```python
from build123d import *

# Parameters (mm, degrees)
SKETCH1_W                                           = 260
SKETCH1_H                                           = 190
BOSS_EXTRUDE1_DEPTH                                 = 40
SKETCH2_R                                           = 15
CUT_EXTRUDE1_DEPTH                                  = 166.90660023
SKETCH3_R                                           = 5.05
CUT_EXTRUDE2_DEPTH                                  = 166.90660023
SKETCH4_R                                           = 9.770548986
CUT_EXTRUDE3_DEPTH                                  = 166.90660023
CBORE_FOR_M8_HEX_SOCKET_HEAD_CAP_SCREW1_D           = 8.4
CBORE_FOR_M8_HEX_SOCKET_HEAD_CAP_SCREW1_CBORE_D     = 15
CBORE_FOR_M8_HEX_SOCKET_HEAD_CAP_SCREW1_CBORE_DEPTH = 8.6
F_8_0MM_DOWEL_HOLE1_D                               = 8
F_10_0MM_DOWEL_HOLE1_D                              = 10
SKETCH15_R                                          = 8.5
CUT_EXTRUDE4_DEPTH                                  = 31.9


with BuildPart() as part:
    # Sketch1 → Boss-Extrude1 (new body)
    with BuildSketch(Plane(origin=(0, 0, 0), x_dir=(1, 0, 0), z_dir=(0, 1, 0))):
        Rectangle(SKETCH1_W, SKETCH1_H)
    extrude(amount=-BOSS_EXTRUDE1_DEPTH)

    # Sketch2 → Cut-Extrude1 (cut, through all)
    with BuildSketch(Plane(origin=(0, 0, 0), x_dir=(1, 0, 0), z_dir=(0, 1, 0))):
        with Locations(Location((-90, 55, 0), (0, 0, 270))):
            Circle(SKETCH2_R)
        with Locations(Location((90, 55, 0), (0, 0, 270))):
            Circle(SKETCH2_R)
    extrude(amount=-CUT_EXTRUDE1_DEPTH, mode=Mode.SUBTRACT)

    # Sketch3 → Cut-Extrude2 (cut, through all)
    with BuildSketch(Plane.XZ.offset(40)):
        with Locations(Location((-55, 70, 0), (0, 0, 270))):
            Circle(SKETCH3_R)
        with Locations(Location((55, 70, 0), (0, 0, 270))):
            Circle(SKETCH3_R)
        with Locations(Location((55, -5, 0), (0, 0, 270))):
            Circle(SKETCH3_R)
        with Locations(Location((-55, -5, 0), (0, 0, 270))):
            Circle(SKETCH3_R)
    extrude(amount=-CUT_EXTRUDE2_DEPTH, mode=Mode.SUBTRACT)

    # Sketch4 → Cut-Extrude3 (cut, through all)
    with BuildSketch(Plane.XZ.offset(40)):
        with Locations(Location((0, 32.5, 0), (0, 0, 270))):
            Circle(SKETCH4_R)
    extrude(amount=-CUT_EXTRUDE3_DEPTH, mode=Mode.SUBTRACT)

    # CBORE for M8 Hex Socket Head Cap Screw1 (through all)
    with Locations(Plane(origin=(0, -40, 0), x_dir=(-1, 0, 0), z_dir=(0, -1, 0))):
        with Locations((-49, -11.95), (-49, -53.05), (49, -53.05), (49, -11.95)):
            CounterBoreHole(CBORE_FOR_M8_HEX_SOCKET_HEAD_CAP_SCREW1_D / 2, CBORE_FOR_M8_HEX_SOCKET_HEAD_CAP_SCREW1_CBORE_D / 2, CBORE_FOR_M8_HEX_SOCKET_HEAD_CAP_SCREW1_CBORE_DEPTH)

    # Ø8.0mm Dowel Hole1 (through all)
    with Locations(Plane(origin=(0, -40, 0), x_dir=(-1, 0, 0), z_dir=(0, -1, 0))):
        with Locations((-49, -32.5), (49, -32.5)):
            Hole(F_8_0MM_DOWEL_HOLE1_D / 2)

    # Ø10.0mm Dowel Hole1 (through all)
    with Locations(Plane(origin=(0, -40, 0), x_dir=(-1, 0, 0), z_dir=(0, -1, 0))):
        with Locations((-100, 17.5), (-100, -82.5), (100, -82.5), (100, 17.5)):
            Hole(F_10_0MM_DOWEL_HOLE1_D / 2)

    # Sketch15 → Cut-Extrude4 (cut)
    with BuildSketch(Plane.XZ.offset(40)):
        with Locations(Location((-100, 82.5, 0), (0, 0, 270))):
            Circle(SKETCH15_R)
        with Locations(Location((100, 82.5, 0), (0, 0, 270))):
            Circle(SKETCH15_R)
        with Locations(Location((100, -17.5, 0), (0, 0, 270))):
            Circle(SKETCH15_R)
        with Locations(Location((-100, -17.5, 0), (0, 0, 270))):
            Circle(SKETCH15_R)
    extrude(amount=-CUT_EXTRUDE4_DEPTH, mode=Mode.SUBTRACT)


solid = part.part
```
Build history of the part. All positions in model axes, mm. A direction names the side the tool comes from. Give positions to 0.01 mm unless a question says otherwise; leave off trailing zeros. Order: outer loops, then holes, each group sorted by start corner. A loop starts at its lowest first (then second) coordinate and runs counter-clockwise, first axis right, second up. Notation, with made-up numbers: M 76,9.25 L 84,9.25 A11 ccw 84,30.25 Z; hole C 28,-39 d9. An arc over 180 degrees is marked long. Return JSON: item names as keys, results as strings.
Q1. Wall check: probe 1 along Z at (x, y) = (49, -19.5); probe 2 along X at (y, z) = (-34, 53); probe 3 along X at (y, z) = (-19, 32). Give the ranges that are in metal, low to high. Write a range as from..to.
Answer list:
{"probe 1": "z = -95..7.75, 16.15..28.5, 36.5..48.85, 57.25..95", "probe 2": "x = -130..-56.5, -41.5..41.5, 56.5..130", "probe 3": "x = -130..-52.97, -45.03..-9.76, 9.76..45.03, 52.97..130"}
Q2. Flat gauge pins, fed straight in: pin 1 (7 mm diameter, centred on x = 49, z = 32.5, fed in from +Y); pin 2 (13.5 mm diameter, centred on x = -100, z = -17.5, fed in from -Y); pin 3 (12 mm diameter, centred on x = 48.5, z = 52, fed in from -Y). Where does each tip first touch, or does it go through?
Answer list:
{"pin 1": "passes through", "pin 2": "stops at y = -8.1", "pin 3": "stops at y = -31.4"}
Q3. Band-saw the part on D-D (z = -17.5). Give the cut face in (x, y), then the cut area to 3 significant figures.
Answer list:
{"outline": "M -130,-40 L -108.5,-40 L -108.5,-8.1 L -105,-8.1 L -105,0 L -130,0 Z; M -95,-8.1 L -91.5,-8.1 L -91.5,-40 L 91.5,-40 L 91.5,-8.1 L 95,-8.1 L 95,0 L -95,0 Z; M 105,-8.1 L 108.5,-8.1 L 108.5,-40 L 130,-40 L 130,0 L 105,0 Z", "area": "9,150 mm^2"}
Q4. Band-saw the part on C-C (x = 100). Give the cut face in (y, z).
Answer list:
{"outline": "M -40,-95 L 0,-95 L 0,-66.18 L -40,-66.18 Z; M -40,-43.82 L 0,-43.82 L 0,-22.5 L -8.1,-22.5 L -8.1,-26 L -40,-26 Z; M -40,-9 L -8.1,-9 L -8.1,-12.5 L 0,-12.5 L 0,77.5 L -8.1,77.5 L -8.1,74 L -40,74 Z; M -40,91 L -8.1,91 L -8.1,87.5 L 0,87.5 L 0,95 L -40,95 Z"}
Q5. Band-saw the part on A-A (z = 11.95). Give the cut face in (x, y), then the cut area to 3 significant figures.
Answer list:
{"outline": "M -130,-40 L -56.5,-40 L -56.5,-31.4 L -53.2,-31.4 L -53.2,0 L -130,0 Z; M -44.8,-31.4 L -41.5,-31.4 L -41.5,-40 L 41.5,-40 L 41.5,-31.4 L 44.8,-31.4 L 44.8,0 L -44.8,0 Z; M 53.2,-31.4 L 56.5,-31.4 L 56.5,-40 L 130,-40 L 130,0 L 53.2,0 Z", "area": "9,610 mm^2"}
Q6. Band-saw the part on B-B (y = -13). Count the separate pieces of the cut face and the enclosed holes in it, then the cut area to 3 significant figures.
Answer list:
{"separate pieces": "1", "enclosed holes": "17", "area": "46,100 mm^2"}
Q7. Two-plate mould, pull along Z, no slides. Class faces 1 (the face through (45.8, -31.4, 56.3)), 2 (the face through (-2, 0, -1)), 3 (the face through (-2, -20, -95)): pulls with the +Z half, pulls with the -Z half, needs draft (parallel to the pull), parting line crosses it, or undercut.
Answer list:
{"face 1": "undercut", "face 2": "needs draft", "face 3": "pulls with the -Z half"}
Q8. 3-axis set-ups, long thin cutter, end or side, ignore diameter. For faces 4 (the face through (-130, -20, 1)), 5 (the face through (96, -8.1, 79)): which of +Z, -Z, +X, -X, +Y, -Y reach the whole face in a straight line?
Answer list:
{"face 4": "+Z, -Z, -X, +Y, -Y", "face 5": "-Y"}
